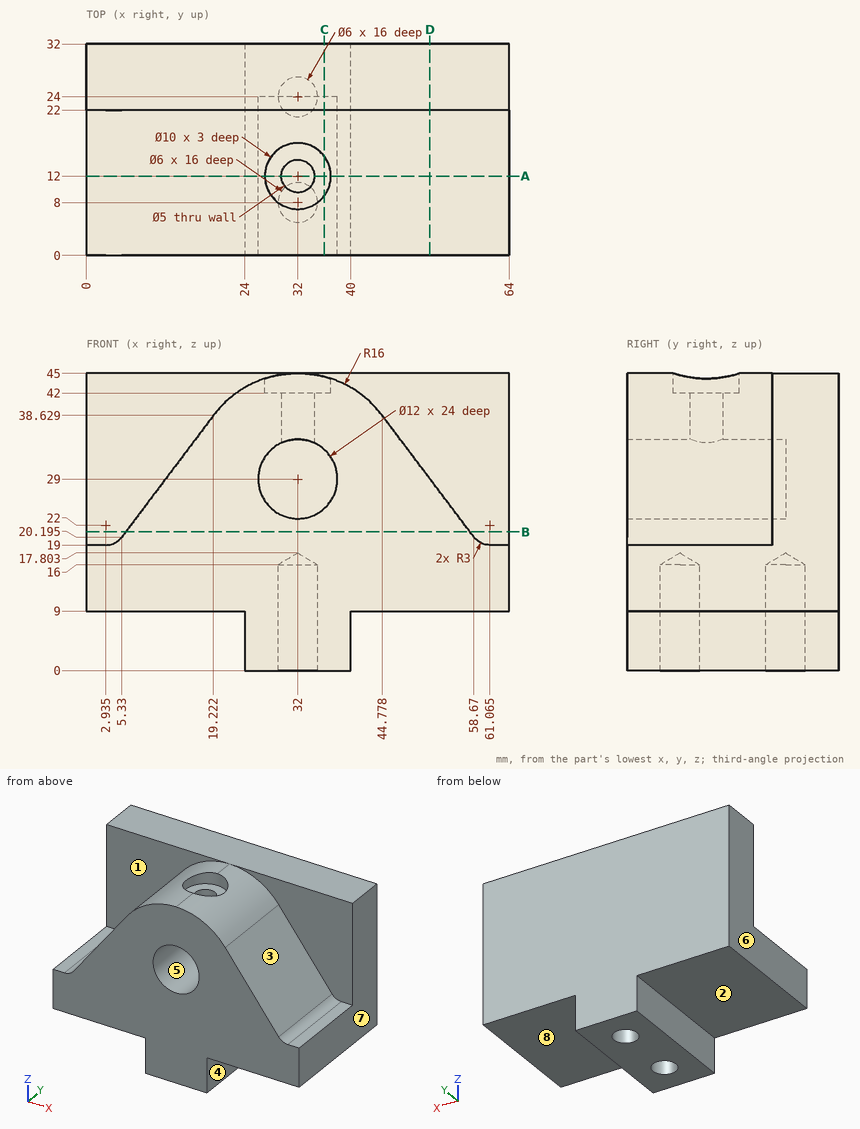
Study the drawing (mm; zero at the part's minimum x, y, z) and answer. A direction names the side the tool comes from. Give positions to 0.01 mm unless a question says otherwise; leave off trailing zeros. Order: outer loops, then holes, each group sorted by start corner. A loop starts at its lowest first (then second) coordinate and runs counter-clockwise, first axis right, second up. Notation, with made-up numbers: (72, -6.5) - (86, -6.5) arc R28 ccw to (86, 23.5) - close; hole circle Ø10 at (11.5, 68). An arc over 180 degrees is marked (long way). Use one line per item in the form item = value. Start each with the question number.
(1) A cutting plane is placed at D-D, the plane x = 52. Write down the section's boundary in (y, z) (1 decimal), then the cut area to 3 significant figures.
(2) A cutting plane is placed at B-B, the plane z = 21. Write down the section's boundary in (x, y).
(3) Flat-ended cylindrical pins translate along their axes: pin 1 Ø21 at (x, z) = (54.5, 28.5) entering from -Y; pin 2 Ø1.5 at (y, z) = (15, 5.5) entering from -X; pin 3 Ø1.5 at (y, z) = (18, 38) entering from +X; pin 4 Ø12 at (x, y) = (46.5, 11.5) entering from -Z. Find the tip coordinate at first contact, or state that the pin passes through.
(4) Consider line 1 (Y direction, x = 32, z = 12); line 2 (Y direction, x = 32, z = 38.5); line 3 (Y direction, x = 6, z = 34.5). Determine where each line is inside the solid, lowest interval first. Write a range as from..to.
(5) The mould has two halves that part along X. Classify the marked faces 5, 6, 7 and 8: released by +X, released by -X, zero draft, split by the parting line, or undercut.
(6) A cutting plane is placed at A-A, the plane y = 12. Write down the section's boundary in (x, z) (1 decimal), then the cut area to 3 significant figures.
(7) A cutting plane is placed at C-C, the plane x = 36. Write down the section's boundary in (y, z).
(8) For the marked faces 1, 2, 3 and 4, determine the directions among +Z, -Z, +X, -X, +Y, -Y from which every point of the face is accessible in a straight line to the end or side of a thin tool.
Ans:
q1.outline = (0, 9) - (32, 9) - (32, 45) - (22, 45) - (22, 29) - (0, 29) - close
q1.area = 801 mm^2
q2.outline = (0, 22) - (5.94, 22) - (5.94, 0) - (58.06, 0) - (58.06, 22) - (64, 22) - (64, 32) - (0, 32) - close
q3.pin_1 = 0
q3.pin_2 = 24
q3.pin_3 = 45.82
q3.pin_4 = 9
q4.line_1 = 0..5, 11..21, 27..32
q4.line_2 = 0..9.5, 14.5..32
q4.line_3 = 22..32
q5.face_5 = undercut
q5.face_6 = released by -X
q5.face_7 = released by +X
q5.face_8 = zero draft
q6.outline = (0, 9) - (24, 9) - (24, 0) - (40, 0) - (40, 9) - (64, 9) - (64, 19) - (61.1, 19) arc R3 cw to (58.7, 20.2) - (44.8, 38.6) arc R16 ccw to (37, 44.2) - (37, 42) - (34.5, 42) - (34.5, 34.5) arc R6 cw (long way) to (29.5, 34.5) - (29.5, 42) - (27, 42) - (27, 44.2) arc R16 ccw to (19.2, 38.6) - (5.3, 20.2) arc R3 cw to (2.9, 19) - (0, 19) - close
q6.area = 1,510 mm^2
q7.outline = (0, 0) - (32, 0) - (32, 45) - (22, 45) - (22, 44.49) - (15, 44.49) - (15, 42) - (9, 42) - (9, 44.49) - (0, 44.49) - (0, 33.47) - (24, 33.47) - (24, 24.53) - (0, 24.53) - close
q8.face_1 = +Z, -X, -Y
q8.face_2 = -Z, -X, +Y, -Y
q8.face_3 = +Z, +X, -Y
q8.face_4 = -Z, +X, +Y, -Y
